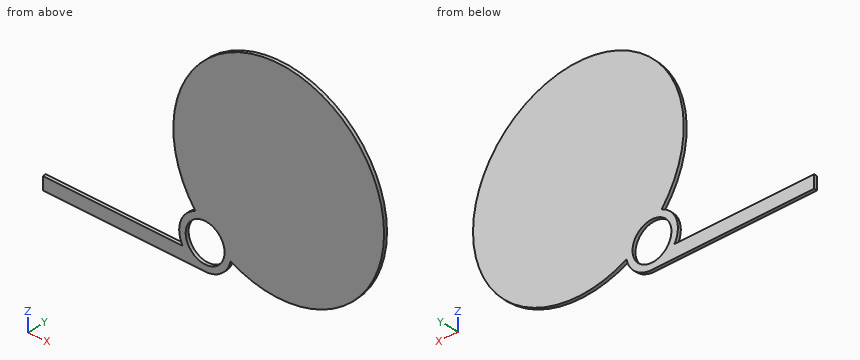
from build123d import *

# Parameters (mm, degrees)
F1_DEPTH = 1


with BuildPart() as f1:
    # F0 (on Front) → F1 (new body)
    with BuildSketch(Plane.XZ):
        with BuildLine():
            ThreePointArc((-14.8566900459, -28.905514368), (16.9323296316, -27.7406959762), (32.5, 0))
            ThreePointArc((32.5, 0), (-10.5130507391, 30.7526545872), (-25.6985085636, -19.8956441868))
            ThreePointArc((-25.6985085636, -19.8956441868), (-18.2250702901, -20.6769291866), (-14.6961524227, -27.3108891325))
            ThreePointArc((-14.6961524227, -27.3108891325), (-14.7363880099, -28.1122320632), (-14.8566900459, -28.905514368))
        make_face()
        with BuildLine():
            ThreePointArc((-14.6961524227, -27.3108891325), (-18.2250702901, -20.6769291866), (-25.6985085636, -19.8956441868))
            ThreePointArc((-25.6985085636, -19.8956441868), (-25.0312995122, -20.7288215953), (-24.3370897754, -21.5396393021))
            ThreePointArc((-24.3370897754, -21.5396393021), (-19.0799129475, -22.5231117715), (-16.6961524227, -27.3108891325))
            ThreePointArc((-16.6961524227, -27.3108891325), (-16.7026347711, -27.5897191161), (-16.7220678093, -27.8679466086))
            ThreePointArc((-16.7220678093, -27.8679466086), (-15.7978993424, -28.4020488058), (-14.8566900459, -28.905514368))
            ThreePointArc((-14.8566900459, -28.905514368), (-14.7363880099, -28.1122320632), (-14.6961524227, -27.3108891325))
        make_face()
        with BuildLine():
            ThreePointArc((-24.3370897754, -21.5396393021), (-25.0312995122, -20.7288215953), (-25.6985085636, -19.8956441868))
            ThreePointArc((-25.6985085636, -19.8956441868), (-30.2612668731, -24.7091506075), (-29.624355653, -31.3108891325))
            Line((-29.624355653, -31.3108891325), (-27.1682883777, -31.3108891325))
            ThreePointArc((-27.1682883777, -31.3108891325), (-28.4591158208, -25.6410828946), (-24.3370897754, -21.5396393021))
        make_face()
        with BuildLine():
            ThreePointArc((-22.6961524227, -35.3108891325), (-17.6343840501, -33.5059275458), (-14.8566900459, -28.905514368))
            ThreePointArc((-14.8566900459, -28.905514368), (-15.7978993424, -28.4020488058), (-16.7220678093, -27.8679466086))
            ThreePointArc((-16.7220678093, -27.8679466086), (-18.6552580203, -31.7461086793), (-22.6961524227, -33.3108891325))
            Line((-22.6961524227, -33.3108891325), (-22.6961524227, -35.3108891325))
        make_face()
        with BuildLine():
            ThreePointArc((-22.6961524227, -35.3108891325), (-26.6961524227, -34.2390923627), (-29.624355653, -31.3108891325))
            Line((-29.624355653, -31.3108891325), (-72.6961524227, -31.3108891325))
            Line((-72.6961524227, -31.3108891325), (-72.6961524227, -35.3108891325))
            Line((-72.6961524227, -35.3108891325), (-22.6961524227, -35.3108891325))
        make_face()
        with BuildLine():
            Line((-27.1682883777, -31.3108891325), (-29.624355653, -31.3108891325))
            ThreePointArc((-29.624355653, -31.3108891325), (-26.6961524227, -34.2390923627), (-22.6961524227, -35.3108891325))
            Line((-22.6961524227, -35.3108891325), (-22.6961524227, -33.3108891325))
            ThreePointArc((-22.6961524227, -33.3108891325), (-25.1456421655, -32.7881147075), (-27.1682883777, -31.3108891325))
        make_face()
    extrude(amount=F1_DEPTH)


solid = f1.part
For this review, take the finished solid that the model builds, in its own axes (mm). Coordinates: 2 decimals unless noted, no trailing zeros. Order: outer loops, then holes, each group sorted by start corner. A loop starts at its lowest first (then second) coordinate and runs counter-clockwise, first axis right, second up. Notation, with made-up numbers: (22, 37) -> (73, 37) arc R27 cw to (73, 69) -> close; hole circle Ø9 at (-3, -5.75). An arc over 180 degrees is marked (long way). Return JSON: item names as keys, results as strings.
1. We need section B-B on z = 16.5. Write out the cut boundary in (x, y), and give its area (3 significant figures).
Answer block:
{"outline": "(-28, -1) -> (28, -1) -> (28, 0) -> (-28, 0) -> close", "area": "56.0 mm²"}
2. For line 1 (Z direction, x = -62, y = -0.1); line 2 (Z direction, x = -29, y = -0.15); line 3 (Z direction, x = -21.5, y = -0.7), list the stretches that pass through material, from the lowest coordinate up. Write a range as from..to.
Answer block:
{"line 1": "-35.31..-31.31", "line 2": "-35.31..-22.39, -14.67..14.67", "line 3": "-35.22..-33.19, -21.43..24.37"}
3. We need section C-C on x = 0. Write out the cut boundary in (y, z).
Answer block:
{"outline": "(-1, -32.5) -> (0, -32.5) -> (0, 32.5) -> (-1, 32.5) -> close"}
4. We need section A-A on y = -0.3. Write out the cut boundary in (x, z).
Answer block:
{"outline": "(-72.7, -35.31) -> (-22.7, -35.31) arc R8 ccw to (-14.86, -28.91) arc R32.5 ccw (long way) to (-25.7, -19.9) arc R8 ccw to (-29.62, -31.31) -> (-72.7, -31.31) -> close; hole circle Ø12 at (-22.7, -27.31)"}
